Could you check a few things on this model? Use its own coordinates, in mm. A direction names the side the tool comes from. Round coordinates to 2 decimals unless told otherwise and drop trailing zeros. Write each loop counter-clockwise with the first axis right and the second up, starting at its lowest first coordinate (ties: lowest second). Pieces come first, ordered by that corner, then holes. Notation, with made-up numbers: (47.25, 84.5) -> (61.25, 84.5) arc R31 ccw to (61.25, 118.5) -> close; hole circle Ø3 at (-30.75, 14.25). An arc over 180 degrees is marked (long way). One line per question, with ' | ' between items. Start each with the question number.
1. Imagine slicing it at D-D, the plane x = 31. List the corners of the cut face in (y, z) for me (3 decimals), and give its area (3 significant figures).
2. For pin 1 Ø6 at (x, y) = (32, 3) entering from +Z (3 decimals); pin 2 Ø10 at (x, z) = (27.5, 11) entering from +Y, each with a flat end and sliding along its axis, tell me the tip position at first contact or that it passes through.
3. Imagine slicing it at B-B, the plane y = 0. List the corners of the cut face in (x, z) for me (3 decimals), and give its area (3 significant figures).
4. Imagine slicing it at A-A, the plane x = 75. List the corners of the cut face in (y, z) for me (3 decimals), and give its area (3 significant figures).
5. For faces 1 (the flat face through (87.7, -13, 8)), 2 (the flat face through (37, -12.7, 16)), which set-ups out of +Z, -Z, +X, -X, +Y, -Y let a thin tool reach every point of the face, with its end or its side?
6. Imagine slicing it at C-C, the plane z = 15. List the corners of the cut face in (x, y) for me (3 decimals), and give its area (3 significant figures).
7. If I drill on line 1 along Y through (x, z) = (75, 2.55) (3 decimals); line 2 along X through (y, z) = (1.75, 1.75); line 3 along Z through (x, y) = (29.5, -5) (3 decimals), over which ranges is the centre line in solid material (lowest first)? Write a range as [from, to].
from build123d import *

# Parameters (mm, degrees)
SKETCH1_W           = 100.4
SKETCH1_H           = 28.575
SKETCH1_R           = 3.175
BOSS_EXTRUDE1_DEPTH = 3.175
SKETCH2_W           = 100.4
SKETCH2_H           = 3.175
BOSS_EXTRUDE2_DEPTH = 25.4


with BuildPart() as part:
    # Sketch1 → Boss-Extrude1 (new body)
    with BuildSketch(Plane.XY):
        with Locations((37.5, -1.5875)):
            Rectangle(SKETCH1_W, SKETCH1_H)
        Circle(SKETCH1_R, mode=Mode.SUBTRACT)
        with Locations((75, 0)):
            Circle(SKETCH1_R, mode=Mode.SUBTRACT)
    extrude(amount=BOSS_EXTRUDE1_DEPTH)

    # Sketch2 → Boss-Extrude2 (add)
    with BuildSketch(Plane.XY.offset(3.175)):
        with Locations((37.5, -14.2875)):
            Rectangle(SKETCH2_W, SKETCH2_H)
    extrude(amount=BOSS_EXTRUDE2_DEPTH)


solid = part.part
Geometry results:
1) outline: (-15.875, 0) -> (12.7, 0) -> (12.7, 3.175) -> (-12.7, 3.175) -> (-12.7, 28.575) -> (-15.875, 28.575) -> close | area: 171 mm2
2) pin 1: stops at z = 3.175 | pin 2: stops at y = -12.7
3) outline: (-12.7, 0) -> (-3.175, 0) -> (-3.175, 3.175) -> (-12.7, 3.175) -> close; (3.175, 0) -> (71.825, 0) -> (71.825, 3.175) -> (3.175, 3.175) -> close; (78.175, 0) -> (87.7, 0) -> (87.7, 3.175) -> (78.175, 3.175) -> close | area: 278 mm2
4) outline: (-15.875, 0) -> (-3.175, 0) -> (-3.175, 3.175) -> (-12.7, 3.175) -> (-12.7, 28.575) -> (-15.875, 28.575) -> close; (3.175, 0) -> (12.7, 0) -> (12.7, 3.175) -> (3.175, 3.175) -> close | area: 151 mm2
5) face 1: +Z, -Z, +X, +Y, -Y | face 2: +Z, +X, -X, +Y
6) outline: (-12.7, -15.875) -> (87.7, -15.875) -> (87.7, -12.7) -> (-12.7, -12.7) -> close | area: 319 mm2
7) line 1: y = [-15.875, -3.175], [3.175, 12.7] | line 2: x = [-12.7, -2.65], [2.65, 72.35], [77.65, 87.7] | line 3: z = [0, 3.175]
